For this review, take the finished solid that the model builds, in its own axes (mm). Face numbers are marked on the shaded views. A direction names the side the tool comes from. Coordinates: 2 decimals unless noted, no trailing zeros. Order: outer loops, then holes, each group sorted by start corner. A loop starts at its lowest first (then second) coordinate and runs counter-clockwise, first axis right, second up. Notation, with made-up numbers: M -16.5,76.5 L 20.5,76.5 A25 ccw 20.5,109.5 Z; hole C 85.25,54.25 d7. An arc over 180 degrees is marked long. Use CSV: the item, a comma, the result in double quotes.
```python
from build123d import *

# Parameters (mm, degrees)
BOSS_EXTRUDE1_DEPTH = 236
SKETCH5_R           = 1.075
CUT_EXTRUDE1_DEPTH  = 85
FILLET1_R           = 2
SKETCH7_W           = 10
SKETCH7_H           = 236
BOSS_EXTRUDE2_DEPTH = 100
BOSS_EXTRUDE3_DEPTH = 30


with BuildPart() as part:
    # Sketch2 → Boss-Extrude1 (new body)
    with BuildSketch(Plane.XY):
        Polygon((0, 0), (0, 22.212686922), (-10, 22.212686922), (-10, -24.787313078), (171.2, -24.787313078), (171.2, -6.387313078), (19.2, -6.387313078), (19.2, -14.787313078), (0, -14.787313078), align=None)
    extrude(amount=BOSS_EXTRUDE1_DEPTH)

    # Sketch5 → Cut-Extrude1 (cut, symmetric)
    with BuildSketch(Plane(origin=(0, 0, 0), x_dir=(0, 0, -1), z_dir=(1, 0, 0))):
        with Locations(Location((-10, 2.212686922, 0), (0, 0, 90))):
            Circle(SKETCH5_R)
        with Locations(Location((-45.2, 2.212686922, 0), (0, 0, 90))):
            Circle(SKETCH5_R)
        with Locations(Location((-55.2, 2.212686922, 0), (0, 0, 90))):
            Circle(SKETCH5_R)
        with Locations(Location((-90.4, 2.212686922, 0), (0, 0, 90))):
            Circle(SKETCH5_R)
        with Locations(Location((-100.4, 2.212686922, 0), (0, 0, 90))):
            Circle(SKETCH5_R)
        with Locations(Location((-135.6, 2.212686922, 0), (0, 0, 90))):
            Circle(SKETCH5_R)
        with Locations(Location((-145.6, 2.212686922, 0), (0, 0, 90))):
            Circle(SKETCH5_R)
        with Locations(Location((-180.8, 2.212686922, 0), (0, 0, 90))):
            Circle(SKETCH5_R)
        with Locations(Location((-190.8, 2.212686922, 0), (0, 0, 90))):
            Circle(SKETCH5_R)
        with Locations(Location((-226, 2.212686922, 0), (0, 0, 90))):
            Circle(SKETCH5_R)
    extrude(amount=CUT_EXTRUDE1_DEPTH, both=True, mode=Mode.SUBTRACT)

    # Fillet1
    fillet1_edges = [part.edges().sort_by_distance(p)[0] for p in [
        (0, -14.787313078, 118),
        (19.2, -14.787313078, 118),
        (19.2, -6.387313078, 118),
    ]]
    fillet(fillet1_edges, radius=FILLET1_R)

    # Sketch7 → Boss-Extrude2 (add)
    with BuildSketch(Plane(origin=(0, -6.387313078, 0), x_dir=(1, 0, 0), z_dir=(0, 1, 0))):
        with Locations((166.2, -118)):
            Rectangle(SKETCH7_W, SKETCH7_H)
    extrude(amount=-BOSS_EXTRUDE2_DEPTH)

    # Sketch8 → Boss-Extrude3 (add)
    with BuildSketch(Plane(origin=(171.2, 0, 0), x_dir=(0, 0, -1), z_dir=(1, 0, 0))):
        Polygon((-236, -24.787313078), (-236, -30.148189832), (-38.862071019, -106.387313078), (-25, -106.387313078), align=None)
    extrude(amount=BOSS_EXTRUDE3_DEPTH)


solid = part.part
```
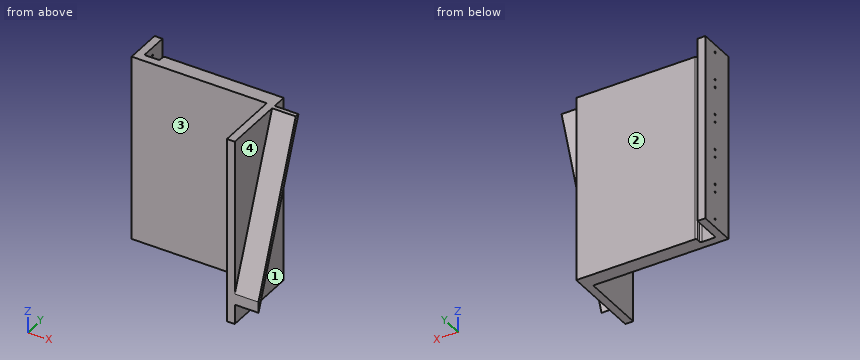
Item 1: Add section D-D on y = -56.5. State the section outline as (x, z) points.
Solutions:
outline,"M 161.2,0 L 171.2,0 L 171.2,154 L 201.2,154 L 201.2,167.86 L 171.2,167.86 L 171.2,236 L 161.2,236 Z"
Item 2: Add section B-B on z = 210.5. State the section outline as (x, y) points, and give its area (3 significant figures).
Solutions:
outline,"M -10,-24.79 L 161.2,-24.79 L 161.2,-106.39 L 171.2,-106.39 L 171.2,-40.01 L 201.2,-40.01 L 201.2,-34.65 L 171.2,-34.65 L 171.2,-6.39 L 21.2,-6.39 A2 ccw 19.2,-8.39 L 19.2,-12.79 A2 cw 17.2,-14.79 L 2,-14.79 A2 cw 0,-12.79 L 0,22.21 L -10,22.21 Z"
area,"4,440 mm^2"
Item 3: For the marked faces 1, 2, 3 and 4, list the 3-axis set-ups (+Z, -Z, +X, -X, +Y, -Y) from which the entire face can be reached by the end or side of a thin tool; tool diameter is ignored.
Solutions:
face 1,"-Z, +X, +Y"
face 2,"+Z, -Z, +X, +Y"
face 3,"+Z, -Z, -X, -Y"
face 4,"+Z, +X, -Y"
Item 4: Clearance check with flat-ended pins moving along their axes: pin 1 Ø12 at (x, z) = (13, 88) entering from +Y; pin 2 Ø1.5 at (x, z) = (101.5, 58) entering from -Y; pin 3 Ø3 at (y, z) = (-3.5, 138) entering from +X; pin 4 Ø2.5 at (y, z) = (2.21, 90.4) entering from -X. State where each tip first meets the part, or that it passes through.
Solutions:
pin 1,"y = -13.66"
pin 2,"y = -24.79"
pin 3,"x = 0"
pin 4,"x = -10"
Item 5: Add section C-C on x = 14. State the section outline as (y, z) points, and give its area (3 significant figures).
Solutions:
outline,"M -24.79,0 L -14.79,0 L -14.79,236 L -24.79,236 Z"
area,"2,360 mm^2"
Item 6: Add section A-A on y = -19. State the section outline as (x, z) points, and give its area (3 significant figures).
Solutions:
outline,"M -10,0 L 171.2,0 L 171.2,236 L -10,236 Z"
area,"42,800 mm^2"
Item 7: To check wall thickness, follow line 1 along X through (y, z) = (-9.5, 157.5); line 2 along Y through (x, z) = (-7.5, 135.6); line 3 along X through (y, z) = (-73, 224.5). State the ranges of each line that lie inside material, in increasing order. Write a range as [from, to].
Solutions:
line 1,"[-10, 0], [19.2, 171.2]"
line 2,"[-24.79, 1.14], [3.29, 22.21]"
line 3,"[161.2, 171.2]"
